For this review, take the finished solid that the model builds, in its own axes (mm). Round coordinates to 2 decimals unless told otherwise and drop trailing zeros. Loops run counter-clockwise (first coordinate to the right, second up) from the corner with the lowest first, then second, coordinate; pieces in that order, holes last. Notation, with made-up numbers: (12.5, 43) -> (50.5, 43) arc R27 ccw to (50.5, 62) -> close; hole circle Ø7 at (46, -4.5). An arc over 180 degrees is marked (long way). Write each question's results on one line, items separated by ' | '.
```python
from build123d import *

# Parameters (mm, degrees)
SKETCH1_R               = 15
SKETCH1_R_2             = 2.2
SKETCH1_R_3             = 1.5
BOSS_EXTRUDE1_DEPTH     = 5
SKETCH2_R               = 6.5
SKETCH2_R_2             = 2.2
BOSS_EXTRUDE2_DEPTH     = 4
BOSS_EXTRUDE3_DEPTH     = 4
SKETCH3_W               = 6
SKETCH3_H               = 2.5
CUT_EXTRUDE1_DEPTH      = 24.043437244
SKETCH5_R               = 1.25
CUT_EXTRUDE2_DEPTH      = 7
SKETCH6_W               = 9
SKETCH6_H               = 2.5
BOSS_EXTRUDE4_DEPTH     = 6
CUT_EXTRUDE3_START      = -4
CUT_EXTRUDE3_DEPTH      = 4
CUT_EXTRUDE4_DEPTH      = 2
CUT_EXTRUDE4_DEPTH_BACK = 14
SKETCH8_R               = 1.25
SKETCH9_R               = 15
CUT_EXTRUDE5_DEPTH      = 2


with BuildPart() as part:
    # Sketch1 → Boss-Extrude1 (new body)
    with BuildSketch(Plane.XY):
        Circle(SKETCH1_R)
        Circle(SKETCH1_R_2, mode=Mode.SUBTRACT)
        with Locations((0, 10)):
            Circle(SKETCH1_R_3, mode=Mode.SUBTRACT)
        with Locations((8.660254038, -5)):
            Circle(SKETCH1_R_3, mode=Mode.SUBTRACT)
        with Locations((-8.660254038, -5)):
            Circle(SKETCH1_R_3, mode=Mode.SUBTRACT)
    extrude(amount=BOSS_EXTRUDE1_DEPTH)

    # Sketch2 → Boss-Extrude2 (add)
    with BuildSketch(Plane.XY.offset(5)):
        Circle(SKETCH2_R)
        Circle(SKETCH2_R_2, mode=Mode.SUBTRACT)
    extrude(amount=BOSS_EXTRUDE2_DEPTH)

    # Sketch4 → Boss-Extrude3 (add)
    with BuildSketch(Plane.XY.offset(5)):
        with BuildLine():
            Line((-4.5, 7.69041576), (-4.5, 4.69041576))
            ThreePointArc((-4.5, 4.69041576), (0, 6.5), (4.5, 4.69041576))
            Line((4.5, 4.69041576), (4.5, 7.69041576))
            Line((4.5, 7.69041576), (-4.5, 7.69041576))
        make_face()
    extrude(amount=BOSS_EXTRUDE3_DEPTH)

    # Sketch3 → Cut-Extrude1 (cut, through all)
    with BuildSketch(Plane.XY.offset(9)):
        with Locations((0, 4.35)):
            Rectangle(SKETCH3_W, SKETCH3_H)
    extrude(amount=-CUT_EXTRUDE1_DEPTH, mode=Mode.SUBTRACT)

    # Sketch5 → Cut-Extrude2 (cut)
    with BuildSketch(Plane(origin=(0, 7.69041576, 0), x_dir=(1, 0, 0), z_dir=(0, 1, 0))):
        with Locations(Location((0, -7, 0), (0, 0, 270))):
            Circle(SKETCH5_R)
    extrude(amount=-CUT_EXTRUDE2_DEPTH, mode=Mode.SUBTRACT)

    # Sketch6 → Boss-Extrude4 (add)
    with BuildSketch(Plane(origin=(-3, 0, 0), x_dir=(0, 0, -1), z_dir=(1, 0, 0))):
        with Locations((-4.5, 4.35)):
            Rectangle(SKETCH6_W, SKETCH6_H)
    extrude(amount=BOSS_EXTRUDE4_DEPTH)

    # Sketch7 → Cut-Extrude3 (cut)
    with BuildSketch(Plane.XY.offset(9).offset(CUT_EXTRUDE3_START)):
        with BuildLine():
            ThreePointArc((-4.5, 4.69041576), (0, 6.5), (4.5, 4.69041576))
            Line((4.5, 4.69041576), (4.5, 7.69041576))
            Line((4.5, 7.69041576), (-4.5, 7.69041576))
            Line((-4.5, 7.69041576), (-4.5, 4.69041576))
        make_face()
    extrude(amount=CUT_EXTRUDE3_DEPTH, mode=Mode.SUBTRACT)

    # Sketch8 → Cut-Extrude4 (cut, two sides: drawn at the far end of the back side and taken through both)
    with BuildSketch(Plane(origin=(0, 5.6, 0), x_dir=(1, 0, 0), z_dir=(0, 1, 0)).offset(-CUT_EXTRUDE4_DEPTH_BACK)):
        with Locations(Location((0, -7, 0), (0, 0, 270))):
            Circle(SKETCH8_R)
    extrude(amount=CUT_EXTRUDE4_DEPTH + CUT_EXTRUDE4_DEPTH_BACK, mode=Mode.SUBTRACT)

    # Sketch9 → Cut-Extrude5 (cut)
    with BuildSketch(Plane(origin=(0, 0, 0), x_dir=(-1, 0, 0), z_dir=(0, 0, -1))):
        Circle(SKETCH9_R)
    extrude(amount=-CUT_EXTRUDE5_DEPTH, mode=Mode.SUBTRACT)


solid = part.part
```
1. Consider section D-D (y = 10). State the section outline as (x, z) points, plus the area to 3 significant figures.
Values found:
outline: (-11.18, 2) -> (-1.5, 2) -> (-1.5, 5) -> (-11.18, 5) -> close; (1.5, 2) -> (11.18, 2) -> (11.18, 5) -> (1.5, 5) -> close | area: 58.1 mm2
2. Draft analysis for pull direction X (two halves, no side actions). For faces 1 (the face through (-14.985, 0.66, 3.479)), 2 (the face through (3, -6, 5)), 3 (the face through (0.05, -4.19, 5.75)), state which applies: released by +X, released by -X, zero draft, split by the parting line, or undercut.
Values found:
face 1: split by the parting line | face 2: zero draft | face 3: undercut
3. Consider section B-B (y = -4.5). State the section outline as (x, z) points.
Values found:
outline: (-14.31, 2) -> (-10.07, 2) -> (-10.07, 5) -> (-14.31, 5) -> close; (-7.25, 2) -> (7.25, 2) -> (7.25, 5) -> (4.69, 5) -> (4.69, 9) -> (-4.69, 9) -> (-4.69, 5) -> (-7.25, 5) -> close; (10.07, 2) -> (14.31, 2) -> (14.31, 5) -> (10.07, 5) -> close; hole circle Ø2.5 at (0, 7)
4. To check wall thickness, follow probe 1 along Y at (x, z) = (0, 3.4); probe 2 along X at (y, z) = (0, 6.25); probe 3 along Z at (x, y) = (0, 4.2). State the ranges of each line that lie inside material, in increasing order.
Values found:
probe 1: y = -15 to -2.2, 2.2 to 8.5, 11.5 to 15 | probe 2: x = -6.5 to -2.2, 2.2 to 6.5 | probe 3: z = 2 to 5.75, 8.25 to 9
5. Consider section A-A (x = 0). State the section outline as (y, z) points, plus the area to 3 significant figures.
Values found:
outline: (-15, 2) -> (-2.2, 2) -> (-2.2, 5.75) -> (-6.5, 5.75) -> (-6.5, 5) -> (-15, 5) -> close; (-6.5, 8.25) -> (-2.2, 8.25) -> (-2.2, 9) -> (-6.5, 9) -> close; (2.2, 2) -> (8.5, 2) -> (8.5, 5) -> (6.5, 5) -> (6.5, 5.75) -> (2.2, 5.75) -> close; (2.2, 8.25) -> (6.5, 8.25) -> (6.5, 9) -> (2.2, 9) -> close; (11.5, 2) -> (15, 2) -> (15, 5) -> (11.5, 5) -> close | area: 80.7 mm2
6. For pin 1 (1.5 mm diameter, centred on x = 0, z = 7, fed in from -Y); pin 2 (4 mm diameter, centred on x = 0, y = 10, fed in from +Z), all flat-tipped, find the tip position at first contact; note any pin that passes through.
Values found:
pin 1: passes through | pin 2: stops at z = 5
7. Consider section C-C (z = 4.25). State the section outline as (x, y) points.
Values found:
outline: circle Ø30 at (0, 0); hole circle Ø3 at (-8.66, -5); hole circle Ø4.4 at (0, 0); hole circle Ø3 at (0, 10); hole circle Ø3 at (8.66, -5)
